Geometry: final body of the model. Coordinates: model frame, mm. Round coordinates to 2 decimals unless told otherwise and drop trailing zeros. Loops run counter-clockwise (first coordinate to the right, second up) from the corner with the lowest first, then second, coordinate; pieces in that order, holes last. Notation, with made-up numbers: (59, -29) - (101, -29) arc R23 cw to (101, 6) - close; hole circle Ø9 at (-1.75, -19). An arc over 180 degrees is marked (long way). Answer as a JSON object with one key per item and string values. Group by question number.
Item 1: Line query: line 1 (Y direction, x = 0.1, z = -0.75); line 2 (X direction, y = -1.05, z = -3.75); line 3 (X direction, y = 0.85, z = -3). Output: solid intervals per line, ascending.
Item 2: First-contact query: pin 1 (3 mm diameter, centred on y = 0.5, z = 1, fed in from -X); pin 2 (1.5 mm diameter, centred on y = 0.5, z = 3, fed in from +X). Flat tips, straight axial feed; report the tip coordinate or a pass-through.
Item 3: Section C-C (z = -2.5). Return the cut outline in (x, y), plus the area to 3 significant figures.
Autodesk Inventor part; units mm, degrees
ref_plane "YZ Plane" through (0, 0, 0) normal (1, 0, 0) x (0, 1, 0)
ref_plane "XZ Plane" through (0, 0, 0) normal (0, 1, 0) x (-1, 0, 0)
ref_plane "XY Plane" through (0, 0, 0) normal (0, 0, 1) x (1, 0, 0)
sketch "スケッチ1" plane through (0, 0, 0) normal (0, 0, 1) x (1, 0, 0)
  circle A0 centre (0, 0) radius 1.5
  dimension "d0" = 3
extrude "押し出し1" add sketch "スケッチ1" along normal blind 6
sketch "スケッチ2" plane through (0, 0, 6) normal (0, 0, 1) x (1, 0, 0)
  circle A0 centre (0, 0) radius 1.5
  circle A1 centre (0, 0) radius 3
  dimension "d3" = 6
extrude "押し出し2" add sketch "スケッチ2" along normal blind 1.75 contours A0 | A1
thread "ねじ1"
chamfer "面取り1" distance 1.5 angle 45 1 edges at (-3, 0, 6)
sketch "スケッチ4" plane through (0, 0, 0) normal (0, 0, -1) x (-1, 0, 0)
  circle A0 centre (0, 0) radius 1.5
extrude "押し出し4" add sketch "スケッチ4" along normal blind 4
sketch "スケッチ5" plane through (0, 0, -4) normal (0, 0, -1) x (-1, 0, 0)
  circle A0 centre (0, 0) radius 1.5
extrude "押し出し5" cut sketch "スケッチ5" against normal blind 2
sketch "スケッチ6" plane through (0, 0, -2) normal (0, 0, -1) x (-1, 0, 0)
  circle A0 centre (0, 0) radius 1.5
extrude "押し出し6" add sketch "スケッチ6" along normal blind 5.25
properties part number "SB　15mm皿ネジ" material "Steel, Mild"
Values:
{
 "1": {"line 1": "y = -1.5 to 1.5", "line 2": "x = -1.07 to 1.07", "line 3": "x = -1.24 to 1.24"},
 "2": {"pin 1": "stops at x = -1.5", "pin 2": "stops at x = 1.5"},
 "3": {"outline": "circle Ø3 at (0, 0)", "area": "7.07 mm^2"}
}
